Part model, mm, in its own coordinate system. A direction names the side the tool comes from. Coordinates: 2 decimals unless noted, no trailing zeros. Write each loop counter-clockwise with the first axis right and the second up, starting at its lowest first coordinate (ties: lowest second). Pieces come first, ordered by that corner, then holes. Notation, with made-up numbers: M 44.5,-17 L 53.5,-17 A27 cw 53.5,8 Z; hole C -20.75,60.5 d8. An arc over 180 degrees is marked long. Use a Markdown table: item, result. Add a question column.
Q1. Mould opens along Y. For faces 1 (the flat face through (-1, 1, -6)), 2 (the cylindrical face through (-68.289, -45.696, 0.084)), 3 (the cylindrical face through (-65.8, -27.4, 0.1)), 4 (the cylindrical face through (68.196, 45.789, -0.084)) say: released by +Y, released by -Y, zero draft, split by the parting line, or undercut.
Q2. Tool access for faces 5 (the cylindrical face through (65.8, -27.6, 0.1)), 6 (the flat face through (-3, 22, -0.8)): list every direction of +Z, -Z, +X, -X, +Y, -Y with a clear straight run to the whole face (end or side of a thin tool).
Q3. Slice it at D-D on x = 0. Write the cut outline in (y, z), then the cut area to 3 significant figures.
Q4. Slice it at B-B on y = -27.5. Write the cut outline in (x, z).
Q5. Wall check: L1, parallel to Y at x = -9.5, z = 4.5; L2, parallel to Y at x = -17.5, z = 3.5; L3, parallel to Y at x = -62.5, z = -0.5. Give the ranges that are in metal, low to high. Write a range as from..to.
Q6. Pin check, flat tips, straight feed: pin 1 Ø7 at (x, y) = (0, 23.5) entering from +Z; pin 2 Ø5.5 at (x, y) = (62.5, -27.5) entering from -Z. Stop position of each tip, or through.
Q7. Slice it at C-C on z = -2.5. Count the separate pieces of the cut face and the enclosed holes in it, then the cut area to 3 significant figures.
Q8. Slice it at A-A on x = 17.5. Write the cut outline in (y, z).
from build123d import *

# Parameters (mm, degrees)
SKETCH1_W           = 140
SKETCH1_H           = 95
BOSS_EXTRUDE1_DEPTH = 6
SKETCH2_R           = 2.75
SKETCH2_R_2         = 3.3
SKETCH2_R_3         = 2.1
CUT_EXTRUDE1_DEPTH  = 86.441500455
SKETCH3_R           = 5.5
CUT_EXTRUDE2_DEPTH  = 6.8
FILLET1_R           = 6


with BuildPart() as part:
    # Sketch1 → Boss-Extrude1 (new, symmetric)
    with BuildSketch(Plane.XY):
        Rectangle(SKETCH1_W, SKETCH1_H)
    extrude(amount=BOSS_EXTRUDE1_DEPTH, both=True)

    # Sketch2 → Cut-Extrude1 (cut, through all)
    with BuildSketch(Plane.XY.offset(6)):
        with Locations((0, 23.5)):
            Circle(SKETCH2_R)
        with Locations((0, -7.5)):
            Circle(SKETCH2_R)
        with Locations((-9.5, 12.5)):
            Circle(SKETCH2_R_2)
        with Locations((-9.5, -27.5)):
            Circle(SKETCH2_R_2)
        with Locations((-17.5, 41.5)):
            Circle(SKETCH2_R)
        with Locations((-40, 41.5)):
            Circle(SKETCH2_R_3)
        with Locations((-64, 41.5)):
            Circle(SKETCH2_R_3)
        with Locations((-62.5, 12.5)):
            Circle(SKETCH2_R_2)
        with Locations((-62.5, -27.5)):
            Circle(SKETCH2_R_2)
        with Locations(Location((62.5, -27.5, 0), (0, 0, 180))):
            Circle(SKETCH2_R_2)
        with Locations(Location((62.5, 12.5, 0), (0, 0, 180))):
            Circle(SKETCH2_R_2)
        with Locations(Location((64, 41.5, 0), (0, 0, 180))):
            Circle(SKETCH2_R_3)
        with Locations(Location((40, 41.5, 0), (0, 0, 180))):
            Circle(SKETCH2_R_3)
        with Locations(Location((17.5, 41.5, 0), (0, 0, 180))):
            Circle(SKETCH2_R)
        with Locations(Location((9.5, -27.5, 0), (0, 0, 180))):
            Circle(SKETCH2_R_2)
        with Locations(Location((9.5, 12.5, 0), (0, 0, 180))):
            Circle(SKETCH2_R_2)
    extrude(amount=-CUT_EXTRUDE1_DEPTH, mode=Mode.SUBTRACT)

    # Sketch3 → Cut-Extrude2 (cut)
    with BuildSketch(Plane.XY.offset(6)):
        with Locations((-9.5, -27.5)):
            Circle(SKETCH3_R)
        with Locations((9.5, -27.5)):
            Circle(SKETCH3_R)
        with Locations((9.5, 12.5)):
            Circle(SKETCH3_R)
        with Locations((0, 23.5)):
            Circle(SKETCH3_R)
        with Locations((-9.5, 12.5)):
            Circle(SKETCH3_R)
    extrude(amount=-CUT_EXTRUDE2_DEPTH, mode=Mode.SUBTRACT)

    # Fillet1
    fillet1_edges = [part.edges().sort_by_distance(p)[0] for p in [
        (-70, 47.5, 0),
        (70, 47.5, 0),
        (70, -47.5, 0),
        (-70, -47.5, 0),
    ]]
    fillet(fillet1_edges, radius=FILLET1_R)


solid = part.part
Recorded:
| question | item | result |
|---|---|---|
| 1 | face 1 | zero draft |
| 1 | face 2 | released by -Y |
| 1 | face 3 | undercut |
| 1 | face 4 | released by +Y |
| 2 | face 5 | +Z, -Z |
| 2 | face 6 | +Z |
| 3 | outline | M -47.5,-6 L -10.25,-6 L -10.25,6 L -47.5,6 Z; M -4.75,-6 L 20.75,-6 L 20.75,-0.8 L 18,-0.8 L 18,6 L -4.75,6 Z; M 26.25,-6 L 47.5,-6 L 47.5,6 L 29,6 L 29,-0.8 L 26.25,-0.8 Z |
| 3 | area | 971 mm² |
| 4 | outline | M -70,-6 L -65.8,-6 L -65.8,6 L -70,6 Z; M -59.2,-6 L -12.8,-6 L -12.8,-0.8 L -15,-0.8 L -15,6 L -59.2,6 Z; M -6.2,-6 L 6.2,-6 L 6.2,-0.8 L 4,-0.8 L 4,6 L -4,6 L -4,-0.8 L -6.2,-0.8 Z; M 12.8,-6 L 59.2,-6 L 59.2,6 L 15,6 L 15,-0.8 L 12.8,-0.8 Z; M 65.8,-6 L 70,-6 L 70,6 L 65.8,6 Z |
| 5 | L1 | -47.5..-33, -22..7, 18..47.5 |
| 5 | L2 | -47.5..38.75, 44.25..47.5 |
| 5 | L3 | -47.5..-30.8, -24.2..9.2, 15.8..40.03, 42.97..47.5 |
| 6 | pin 1 | z = -0.8 |
| 6 | pin 2 | through |
| 7 | separate pieces | 1 |
| 7 | enclosed holes | 16 |
| 7 | area | 12,800 mm² |
| 8 | outline | M -47.5,-6 L 38.75,-6 L 38.75,6 L -47.5,6 Z; M 44.25,-6 L 47.5,-6 L 47.5,6 L 44.25,6 Z |
